Input: part model. Units: mm. Frame: model coordinates. A direction names the side the tool comes from. Coordinates: 2 decimals unless noted, no trailing zeros. Loops run counter-clockwise (first coordinate to the right, second up) from the corner with the lowest first, then second, coordinate; pieces in that order, holes last.
(1) Section B-B, the plane y = 0.6. Return loops of the section in (x, z), then the cut area to 3 significant figures.
(2) Line query: L1, parallel to Z at x = 0.25, y = 3.9; L2, parallel to X at y = 1.4, z = 1.3; L3, parallel to Z at x = 3.25, y = 4.35. Output: solid intervals per line, ascending.
(3) Mould query, pull axis Z, two halves, no side actions, for faces 6 (the face through (-3.093, 2.465, 0.646)), 7 (the face through (-2.5, 4.75, -0.4)), 8 (the face through (0, 2, 2.45)). Classes: released by +Z, released by -Z, zero draft, split by the parting line, or undercut.
(4) Section D-D, the plane z = 0.7. Return loops of the section in (x, y), then the cut area to 3 significant figures.
(5) Contact query for flat-ended pins moving along their axis: P1, Ø0.7, axis at x = 3.5, z = -0.5, coming from the -Y side; P2, Ø0.6, axis at y = 2.5, z = -0.5, coming from the -X side (3 decimals); P3, Ø1, axis at x = 1.5, y = 2.5, coming from the -Z side. Output: stop coordinate, or through.
(6) Section A-A, the plane x = -2.25. Return loops of the section in (y, z), then the cut area to 3 significant figures.
(7) Section C-C, the plane z = -0.5. Return loops of the section in (x, y) (3 decimals).
(8) Set-up query: faces 1 (the face through (3.75, 2, 2)), 2 (the face through (-3.5, 2, 2)), 3 (the face through (-3.75, 2, 2)), 4 (the face through (3.625, 2, 0)), 5 (the face through (-3.625, 2, 0)). Return all of +Z, -Z, +X, -X, +Y, -Y with unobstructed straight access to the full face (end or side cutting, diameter ignored); none if empty.
```python
from build123d import *

# Parameters (mm, degrees)
F1_DEPTH = 5
F4_DEPTH = 0.45
F5_W     = 0.9
F5_H     = 1
F6_DEPTH = 0.25


with BuildPart() as f1:
    # F0 (on Front) → F1 (new body)
    with BuildSketch(Plane.XZ):
        Polygon((-2.8, 0), (0, 0), (2.8, 0), (3.75, 0.95), (3.75, 2.45), (0, 2.45), (-3.75, 2.45), (-3.75, 0.95), align=None)
        Polygon((0, 2.1999999881), (3.4999999881, 2.1999999881), (3.4999999881, 1.0535533955), (2.6964466045, 0.2500000119), (0, 0.2500000119), (-2.6964466045, 0.2500000119), (-3.4999999881, 1.0535533955), (-3.4999999881, 2.1999999881), align=None, mode=Mode.SUBTRACT)
    extrude(amount=-F1_DEPTH)

    # F3 (on offset) → F4 (join, symmetric)
    with BuildSketch(Plane(origin=(0, 2.3, 0), x_dir=(-1, 0, 0), z_dir=(0, 1, 0))):
        Polygon((-3.625, 0.2500000119), (-3.625, -0.7499999881), (-3.375, -0.7499999881), (-3.375, 0), (3.375, 0), (3.375, -0.7499999881), (3.625, -0.7499999881), (3.625, 0.2500000119), align=None)
    extrude(amount=F4_DEPTH, both=True)

    # F5 (on face) → F6 (join)
    with BuildSketch(Plane(origin=(0, 5, 0), x_dir=(-1, 0, 0), z_dir=(0, 1, 0))):
        with Locations((-2.5, -0.2499999881)):
            Rectangle(F5_W, F5_H)
        with Locations((2.5, -0.2499999881)):
            Rectangle(F5_W, F5_H)
    extrude(amount=-F6_DEPTH)


solid = f1.part
```
Report:
1. outline: (-3.75, 0.95) - (-2.8, 0) - (2.8, 0) - (3.75, 0.95) - (3.75, 2.45) - (-3.75, 2.45) - close; hole (-3.5, 1.05) - (-2.7, 0.25) - (2.7, 0.25) - (3.5, 1.05) - (3.5, 2.2) - (-3.5, 2.2) - close
1. area: 4.47 mm2
2. L1: z = 0 to 0.25, 2.2 to 2.45
2. L2: x = -3.75 to -3.5, 3.5 to 3.75
2. L3: z = 0.45 to 0.8, 2.2 to 2.45
3. face 6: undercut
3. face 7: zero draft
3. face 8: released by +Z
4. outline: (-3.5, 0) - (-3.15, 0) - (-3.15, 5) - (-3.5, 5) - close; (3.15, 0) - (3.5, 0) - (3.5, 5) - (3.15, 5) - close
4. area: 3.54 mm2
5. P1: stops at y = 1.85
5. P2: stops at x = -3.625
5. P3: stops at z = 0
6. outline: (0, 0) - (4.75, 0) - (4.75, -0.75) - (5, -0.75) - (5, 0.25) - (0, 0.25) - close; (0, 2.2) - (5, 2.2) - (5, 2.45) - (0, 2.45) - close
6. area: 2.69 mm2
7. outline: (-3.625, 1.85) - (-3.375, 1.85) - (-3.375, 2.75) - (-3.625, 2.75) - close; (-2.95, 4.75) - (-2.05, 4.75) - (-2.05, 5) - (-2.95, 5) - close; (2.05, 4.75) - (2.95, 4.75) - (2.95, 5) - (2.05, 5) - close; (3.375, 1.85) - (3.625, 1.85) - (3.625, 2.75) - (3.375, 2.75) - close
8. face 1: +Z, -Z, +X, +Y, -Y
8. face 2: +Y, -Y
8. face 3: +Z, -Z, -X, +Y, -Y
8. face 4: -Z, +X, +Y, -Y
8. face 5: -Z, -X, +Y, -Y
